Can you work these out from the model? Positions are in its coordinate system, mm. A direction names the side the tool comes from. Give positions to 0.01 mm unless a question says otherwise; leave off trailing zeros. Loops run counter-clockwise (first coordinate to the right, second up) from the corner with the lowest first, then second, coordinate; pieces in that order, holes last. Notation, with made-up numbers: (71.25, 25) - (84.25, 25) arc R21 ccw to (84.25, 46) - close; hole circle Ø8 at (-34, 66.5). An arc over 180 degrees is marked (long way). Use a Markdown table: item, result. Add a question column.
```python
from build123d import *

# Parameters (mm, degrees)
F1_R     = 2.75
F1_R_2   = 1.5
F2_DEPTH = 2
F3_START = 1.5
F3_DEPTH = 0.5
F4_START = 2
F4_DEPTH = 9
F5_SIZE2 = 1.25
F5_SIZE  = 1.25
F6_R     = 0.25


# Not quite as in the source:
# - a feature names something its author has since deleted; it is built from what else it names


with BuildPart() as f2:
    # F1 (on Top) → F2 (new body)
    with BuildSketch(Plane.XY):
        Circle(F1_R)
        Circle(F1_R_2, mode=Mode.SUBTRACT)
        Circle(F1_R_2)
        Polygon((-0.5773502692, -1), (-1.1547005384, 0), (-0.5773502692, 1), (0.5773502692, 1), (1.1547005384, 0), (0.5773502692, -1), align=None, mode=Mode.SUBTRACT)
    extrude(amount=F2_DEPTH)

    # F1 (on Top) → F3 (join)
    with BuildSketch(Plane.XY.offset(F3_START)):
        Polygon((-0.5773502692, 1), (-1.1547005384, 0), (-0.5773502692, -1), (0.5773502692, -1), (1.1547005384, 0), (0.5773502692, 1), align=None)
    extrude(amount=F3_DEPTH)

    # F1 (on Top) → F4 (join)
    with BuildSketch(Plane.XY.offset(F4_START)):
        Circle(F1_R_2)
        Polygon((-0.5773502692, -1), (-1.1547005384, 0), (-0.5773502692, 1), (0.5773502692, 1), (1.1547005384, 0), (0.5773502692, -1), align=None, mode=Mode.SUBTRACT)
        Polygon((-0.5773502692, 1), (-1.1547005384, 0), (-0.5773502692, -1), (0.5773502692, -1), (1.1547005384, 0), (0.5773502692, 1), align=None)
    extrude(amount=F4_DEPTH)

    # F5
    f5_edges = [f2.edges().sort_by_distance(p)[0] for p in [
        (-2.75, 0, 0),
    ]]
    chamfer(f5_edges, length=F5_SIZE, length2=F5_SIZE2)

    # F6
    f6_edges = [f2.edges().sort_by_distance(p)[0] for p in [
        (-2.75, 0, 2),
        (-1.5, 0, 2),
        (-1.5, 0, 0),
        (-2.75, 0, 1.25),
    ]]
    fillet(f6_edges, radius=F6_R)


solid = f2.part
```
1. Suppose I cut it at A-A (z = 4.75). List the corners of the cut face in (x, y) for me.
2. On a 3-axis mill with a long thin cutter (end or side, diameter ignored), from which of +Z, -Z, +X, -X, +Y, -Y can I reach the whole of each face in a straight line? I mean faces 4 (the face through (-1.5, 0.07, 6.56)), 5 (the face through (0, 1, 1)), 6 (the face through (0, 0, 11)). Say none if no direction works.
3. If we mould it in two halves opening along Y, with no side actions, what happens to faces 1 (the face through (-0.596, -2.685, 1.549)), 2 (the face through (1, 2, 2)), 3 (the face through (0.87, -0.49, 0.74))? For each: released by +Y, released by -Y, zero draft, split by the parting line, or undercut.
4. Please list where these lines run through material, in increasing order: line 1 along Z through (x, y) = (0.25, -0.15); line 2 along Y through (x, z) = (0.55, 3.5); line 3 along X through (y, z) = (1.1, 6). Write a range as [from, to].
5. Will this pin go through, and if not, where does the flat tip stop? P1, Ø1.3, axis at x = 0, z = 0.5, coming from the +Y side.
Results below:
| question | item | result |
|---|---|---|
| 1 | outline | circle Ø3 at (0, 0) |
| 2 | face 4 | +Z |
| 2 | face 5 | -Z |
| 2 | face 6 | +Z, +X, -X, +Y, -Y |
| 3 | face 1 | split by the parting line |
| 3 | face 2 | zero draft |
| 3 | face 3 | undercut |
| 4 | line 1 | [1.5, 11] |
| 4 | line 2 | [-1.4, 1.4] |
| 4 | line 3 | [-1.02, 1.02] |
| 5 | P1 | y = 2.65 |
